Work out the finished part from the listing and answer in its coordinate system (mm). A direction names the side the tool comes from. Give positions to 0.01 mm unless a question says otherwise; leave off trailing zeros. Order: outer loops, then holes, each group sorted by start corner. A loop starts at its lowest first (then second) coordinate and runs counter-clockwise, first axis right, second up. Notation, with made-up numbers: (43, 39) -> (71, 39) arc R16 cw to (71, 58) -> close; hole circle Ø4 at (-23, 5). An arc over 180 degrees is marked (long way). Use a Markdown table: item, result. Add a question column.
```python
from build123d import *

# Parameters (mm, degrees)
F0_R     = 38
F1_DEPTH = 50
F2_T     = 2
F3_R     = 12.5
F4_DEPTH = 52.001
F5_R     = 5


with BuildPart() as f1:
    # F0 (on Front) → F1 (new body)
    with BuildSketch(Plane.XZ):
        Circle(F0_R)
    extrude(amount=F1_DEPTH)

    # F2
    f2_openings = [f1.faces().sort_by_distance(p)[0] for p in [
        (0, -50, 0),
    ]]
    offset(amount=F2_T, openings=f2_openings, kind=Kind.INTERSECTION)

    # F3 (on face) → F4 (cut, through all)
    with BuildSketch(Plane(origin=(0, 2, 0), x_dir=(-1, 0, 0), z_dir=(0, 1, 0))):
        Circle(F3_R)
    extrude(amount=-F4_DEPTH, mode=Mode.SUBTRACT)

    # F5
    f5_edges = [f1.edges().sort_by_distance(p)[0] for p in [
        (-40, 2, 0),
    ]]
    fillet(f5_edges, radius=F5_R)


solid = f1.part
```
1) Which of the six approach directions +Z, -Z, +X, -X, +Y, -Y give full straight-line access (tool end or side, diameter ignored) to faces 1 (the cylindrical face through (17.535, -24.65, -33.713)), 2 (the flat face through (0, 2, -15))?
2) Straight lines are drawn through the part: line 1 (Z direction, x = 0, y = -15.5); line 2 (Z direction, x = 0, y = 1); line 3 (Y direction, x = 23, z = 11). For each, find the intervals that lie inside material, in ascending order.
3) The part is cut by section C-C, the plane y = -38. Determine the outline of the cut face in (x, z), then the cut area to 3 significant figures.
4) Determine the mould class of faces 3 (the cylindrical face through (-8.67, -26.17, -39.05)), 4 (the cylindrical face through (-11.923, 1.014, 3.755)), 5 (the flat face through (-9, 0, 9)), 6 (the flat face through (35.4, -50, -14.6)) for opening direction X: released by +X, released by -X, zero draft, split by the parting line, or undercut.
5) The part is cut by section A-A, the plane z = 0. Determine the outline of the cut face in (x, y).
6) The part is cut by section B-B, the plane x = 0. Determine the outline of the cut face in (y, z), then the cut area to 3 significant figures.
7) Flat-ended cylindrical pins translate along their axes: pin 1 (10 mm diameter, centred on x = 2, z = -11, fed in from -Y); pin 2 (6 mm diameter, centred on y = -10, z = 18, fed in from +X); pin 3 (2 mm diameter, centred on x = -25, y = -41, fed in from -Z). Find the tip coordinate at first contact, or state that the pin passes through.
A:
| question | item | result |
|---|---|---|
| 1 | face 1 | -Y |
| 1 | face 2 | +Z, -Z, +X, -X, +Y |
| 2 | line 1 | -40 to -38, 38 to 40 |
| 2 | line 2 | -38 to -12.5, 12.5 to 38 |
| 2 | line 3 | 0 to 2 |
| 3 | outline | circle Ø80 at (0, 0); hole circle Ø76 at (0, 0) |
| 3 | area | 490 mm^2 |
| 4 | face 3 | split by the parting line |
| 4 | face 4 | undercut |
| 4 | face 5 | undercut |
| 4 | face 6 | zero draft |
| 5 | outline | (-40, -50) -> (-38, -50) -> (-38, 0) -> (-12.5, 0) -> (-12.5, 2) -> (-35, 2) arc R5 ccw to (-40, -3) -> close; (12.5, 0) -> (38, 0) -> (38, -50) -> (40, -50) -> (40, -3) arc R5 ccw to (35, 2) -> (12.5, 2) -> close |
| 6 | outline | (-50, -40) -> (-3, -40) arc R5 ccw to (2, -35) -> (2, -12.5) -> (0, -12.5) -> (0, -38) -> (-50, -38) -> close; (-50, 38) -> (0, 38) -> (0, 12.5) -> (2, 12.5) -> (2, 35) arc R5 ccw to (-3, 40) -> (-50, 40) -> close |
| 6 | area | 299 mm^2 |
| 7 | pin 1 | y = 0 |
| 7 | pin 2 | x = 37.08 |
| 7 | pin 3 | z = -32 |
